The figure shows three views and two pictorial views of one solid part (mm, origin at its lowest corner). Answer the questions. Coordinates: 2 decimals unless noted, no trailing zeros. Order: outer loops, then holes, each group sorted by start corner. A loop starts at its lowest first (then second) coordinate and runs counter-clockwise, first axis right, second up. Notation, with made-up numbers: (24.25, 54.25) -> (38.25, 54.25) arc R18 cw to (38.25, 83.25) -> close; hole circle Ø4 at (5.25, -11). An arc over 180 degrees is marked (long way). Return JSON: item names as keys, results as strings.
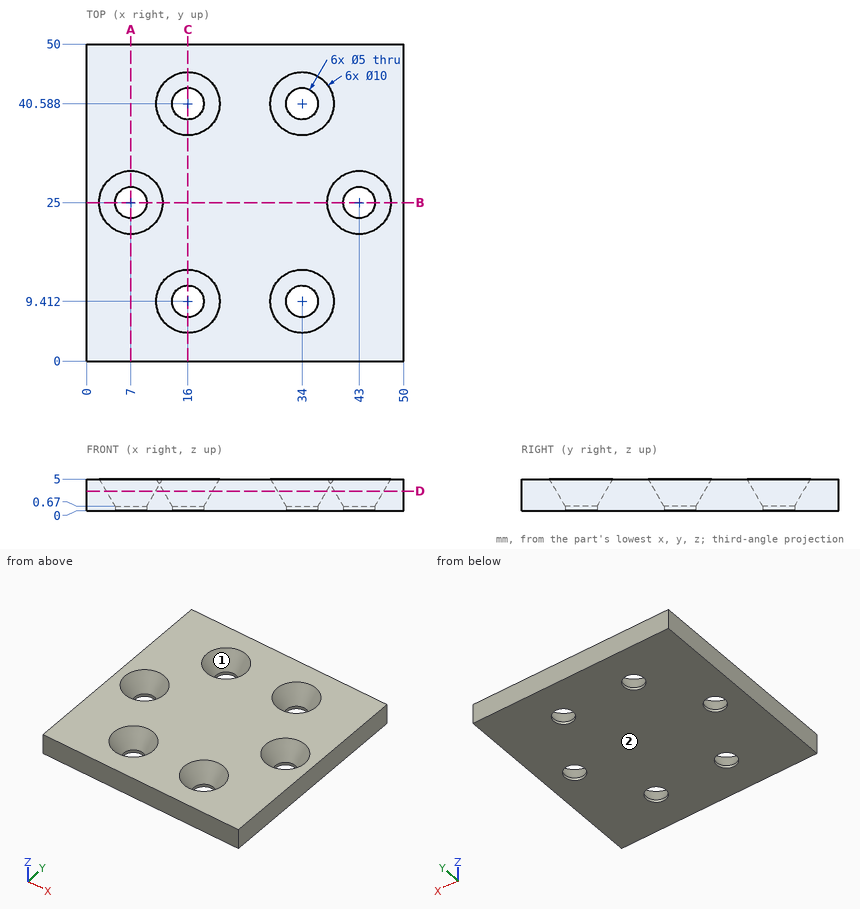
1. The part is cut by section D-D on z = 3.1. Give the vertices of the cut face in (x, y), and give its area (3 significant figures).
Answer block:
{"outline": "(0, 0) -> (50, 0) -> (50, 50) -> (0, 50) -> close; hole circle Ø7.81 at (7, 25); hole circle Ø7.81 at (16, 9.41); hole circle Ø7.81 at (16, 40.59); hole circle Ø7.81 at (34, 9.41); hole circle Ø7.81 at (34, 40.59); hole circle Ø7.81 at (43, 25)", "area": "2,210 mm2"}
2. Determine the mould class of the marked faces 1 and 2 for opening direction X: pulls with the +X half, pulls with the -X half, needs draft (parallel to the pull), parting line crosses it, or undercut.
Answer block:
{"face 1": "undercut", "face 2": "needs draft"}
3. Each of these flat-tipped pins is pushed along its axis until it touches: pin 1 Ø6.5 at (x, y) = (34, 9.41) entering from +Z; pin 2 Ø8 at (x, y) = (34, 40.59) entering from +Z; pin 3 Ø2 at (y, z) = (31, 3.5) entering from -X. Where does it stop, or does it pass through?
Answer block:
{"pin 1": "stops at z = 1.97", "pin 2": "stops at z = 3.27", "pin 3": "stops at x = 0"}
4. The part is cut by section C-C on x = 16. Give the vertices of the cut face in (y, z).
Answer block:
{"outline": "(0, 0) -> (6.91, 0) -> (6.91, 0.67) -> (4.41, 5) -> (0, 5) -> close; (11.91, 0) -> (38.09, 0) -> (38.09, 0.67) -> (35.59, 5) -> (14.41, 5) -> (11.91, 0.67) -> close; (43.09, 0) -> (50, 0) -> (50, 5) -> (45.59, 5) -> (43.09, 0.67) -> close"}
5. The part is cut by section B-B on y = 25. Give the vertices of the cut face in (x, z), and give its area (3 significant figures).
Answer block:
{"outline": "(0, 0) -> (4.5, 0) -> (4.5, 0.67) -> (2, 5) -> (0, 5) -> close; (9.5, 0) -> (40.5, 0) -> (40.5, 0.67) -> (38, 5) -> (12, 5) -> (9.5, 0.67) -> close; (45.5, 0) -> (50, 0) -> (50, 5) -> (48, 5) -> (45.5, 0.67) -> close", "area": "178 mm2"}
6. Consider line 1 (X direction, y = 25, z = 0.5); line 2 (Y direction, x = 34, z = 0.3); line 3 (Y direction, x = 7, z = 0.4). Determine where each line is inside the solid, lowest interval first. Write a range as from..to.
Answer block:
{"line 1": "x = 0..4.5, 9.5..40.5, 45.5..50", "line 2": "y = 0..6.91, 11.91..38.09, 43.09..50", "line 3": "y = 0..22.5, 27.5..50"}
7. The part is cut by section A-A on x = 7. Give the vertices of the cut face in (y, z), and give its area (3 significant figures).
Answer block:
{"outline": "(0, 0) -> (22.5, 0) -> (22.5, 0.67) -> (20, 5) -> (0, 5) -> close; (27.5, 0) -> (50, 0) -> (50, 5) -> (30, 5) -> (27.5, 0.67) -> close", "area": "214 mm2"}
